Geometry: final body of the model. Coordinates: model frame, mm. A direction names the side the tool comes from. Coordinates: 2 decimals unless noted, no trailing zeros. Order: outer loops, then holes, each group sorted by start corner. A loop starts at its lowest first (then second) coordinate and runs counter-clockwise, first axis right, second up. Notation, with made-up numbers: (-18.75, 38.25) - (-8.75, 38.25) arc R16 ccw to (-8.75, 63.25) - close; hole circle Ø3 at (73.5, 56.25). An arc over 180 degrees is marked (long way). Use a Markdown table: item, result. Add a question column.
```python
from build123d import *

# Parameters (mm, degrees)
F0_W     = 107.95
F0_H     = 88.9
F0_W_2   = 101.6
F0_H_2   = 82.55
F0_R     = 3.175
F1_DEPTH = 3.556
F0_R_2   = 1.375
F2_DEPTH = 7.62
F3_DEPTH = 25.4
F4_R     = 3.175
F5_DEPTH = 5.08
F6_R     = 2.54


with BuildPart() as f1:
    # F0 (on Front) → F1 (new body)
    with BuildSketch(Plane.XZ):
        Rectangle(F0_W, F0_H)
        Rectangle(F0_W_2, F0_H_2, mode=Mode.SUBTRACT)
        Rectangle(F0_W_2, F0_H_2)
        with Locations((-38.1, 24.765)):
            Circle(F0_R, mode=Mode.SUBTRACT)
        with Locations((12.7, 24.765)):
            Circle(F0_R, mode=Mode.SUBTRACT)
    extrude(amount=F1_DEPTH)

    # F0 (on Front) → F2 (join)
    with BuildSketch(Plane.XZ):
        with Locations((-38.1, 24.765)):
            Circle(F0_R)
        with Locations((-38.1, 24.765)):
            Circle(F0_R_2, mode=Mode.SUBTRACT)
        with Locations((12.7, 24.765)):
            Circle(F0_R)
        with Locations((12.7, 24.765)):
            Circle(F0_R_2, mode=Mode.SUBTRACT)
    extrude(amount=F2_DEPTH)

    # F0 (on Front) → F3 (join)
    with BuildSketch(Plane.XZ):
        Rectangle(F0_W, F0_H)
        Rectangle(F0_W_2, F0_H_2, mode=Mode.SUBTRACT)
    extrude(amount=F3_DEPTH)

    # F4 (on face) → F5 (cut)
    with BuildSketch(Plane.XY.offset(44.45)):
        with Locations((1.27, -7.62)):
            Circle(F4_R)
        with Locations((-31.75, -7.62)):
            Circle(F4_R)
    extrude(amount=-F5_DEPTH, mode=Mode.SUBTRACT)

    # F6
    f6_edges = [f1.edges().sort_by_distance(p)[0] for p in [
        (-53.975, -12.7, 44.45),
        (-50.8, -14.478, 41.275),
        (53.975, -12.7, 44.45),
        (-53.975, -12.7, -44.45),
        (50.8, -14.478, 41.275),
        (-50.8, -14.478, -41.275),
        (53.975, -12.7, -44.45),
        (50.8, -14.478, -41.275),
        (0, 0, -44.45),
        (53.975, 0, 0),
        (-53.975, 0, 0),
        (0, 0, 44.45),
        (9.525, -3.556, 24.765),
        (-41.275, -3.556, 24.765),
    ]]
    fillet(f6_edges, radius=F6_R)


solid = f1.part
```
1) Set-up query: faces 1 (the face through (-4, -25.4, -43)), 2 (the face through (50.8, -14, -1)). Return all of +Z, -Z, +X, -X, +Y, -Y with unobstructed straight access to the full face (end or side cutting, diameter ignored); none if empty.
2) Pin query (flat end, axial travel): pin 1 (2.5 mm diameter, centred on x = -38.1, z = 24.765, fed in from -Y); pin 2 (1.9 mm diameter, centred on x = -38.5, z = 25.5, fed in from -Y); pin 3 (8 mm diameter, centred on x = -15.5, z = 7.5, fed in from -Y). Return the tip coordinate at first contact, or that it passes through.
3) Ray query, line 1 along Z through (x, y) = (38, -7) (3 decimals); line 2 along X through (y, z) = (-18.5, 38) (3 decimals); line 3 along Y through (x, z) = (1, 42). Return the intervals inside material, ascending.
4) Section D-D (x = -18.5). Return loops of the section in (y, z) (3 decimals), then the cut area to 3 significant figures.
5) Draft query along Z for faces 3 (the face through (0.86, -4.47, 42.88)), 4 (the face through (12.287, -6.847, 27.913)), 5 (the face through (53.211, -13.81, 43.726)), 6 (the face through (-1, -14, -44.45)). Return one class per face: pulls with the +Z half, pulls with the -Z half, needs draft (parallel to the pull), parting line crosses it, or undercut.
6) Section A-A (x = 1.27). Return loops of the section in (y, z) (3 decimals).
7) Section B-B (y = -14). Return loops of the section in (x, z) (3 decimals), then the cut area to 3 significant figures.
8) Section C-C (z = -26). Return loops of the section in (x, y) (3 decimals).
Values follow:
| question | item | result |
|---|---|---|
| 1 | face 1 | +Z, -Z, +X, -X, -Y |
| 1 | face 2 | -Y |
| 2 | pin 1 | passes through |
| 2 | pin 2 | stops at y = -7.62 |
| 2 | pin 3 | stops at y = -3.56 |
| 3 | line 1 | z = -44.45 to -41.275, 41.275 to 44.45 |
| 3 | line 2 | x = -53.975 to -50.8, 50.8 to 53.975 |
| 3 | line 3 | y = -25.4 to -10.78, -4.46 to 0 |
| 4 | outline | (-25.4, -44.45) - (-2.54, -44.45) arc R2.54 ccw to (0, -41.91) - (0, 41.91) arc R2.54 ccw to (-2.54, 44.45) - (-25.4, 44.45) - (-25.4, 41.275) - (-3.556, 41.275) - (-3.556, -41.275) - (-25.4, -41.275) - close |
| 4 | area | 452 mm² |
| 5 | face 3 | needs draft |
| 5 | face 4 | undercut |
| 5 | face 5 | pulls with the +Z half |
| 5 | face 6 | pulls with the -Z half |
| 6 | outline | (-25.4, -44.45) - (-2.54, -44.45) arc R2.54 ccw to (0, -41.91) - (0, 41.91) arc R2.54 ccw to (-2.54, 44.45) - (-4.445, 44.45) - (-4.445, 41.275) - (-3.556, 41.275) - (-3.556, -41.275) - (-25.4, -41.275) - close; (-25.4, 41.275) - (-10.795, 41.275) - (-10.795, 44.45) - (-25.4, 44.45) - close |
| 7 | outline | (-53.975, -41.91) arc R2.54 ccw to (-51.435, -44.45) - (51.435, -44.45) arc R2.54 ccw to (53.975, -41.91) - (53.975, 41.91) arc R2.54 ccw to (51.435, 44.45) - (-51.435, 44.45) arc R2.54 ccw to (-53.975, 41.91) - close; hole (-50.8, -38.735) arc R2.54 ccw to (-48.26, -41.275) - (48.26, -41.275) arc R2.54 ccw to (50.8, -38.735) - (50.8, 38.735) arc R2.54 ccw to (48.26, 41.275) - (-48.26, 41.275) arc R2.54 ccw to (-50.8, 38.735) - close |
| 7 | area | 1,210 mm² |
| 8 | outline | (-53.975, -25.4) - (-50.8, -25.4) - (-50.8, -3.556) - (50.8, -3.556) - (50.8, -25.4) - (53.975, -25.4) - (53.975, -2.54) arc R2.54 ccw to (51.435, 0) - (-51.435, 0) arc R2.54 ccw to (-53.975, -2.54) - close |
